CAD build for the part. Positions are in the model's coordinates, mm. A direction names the side the tool comes from. Coordinates: 2 decimals unless noted, no trailing zeros. Loops run counter-clockwise (first coordinate to the right, second up) from the corner with the lowest first, then second, coordinate; pieces in that order, holes last. Notation, with made-up numbers: (-33.5, 34) -> (20.5, 34) arc R15 ccw to (20.5, 48) -> close; hole circle Ø3 at (60.25, -32.5). An arc over 180 degrees is marked (long way). Return JSON: item names as keys, results as strings. Group by question number.
(1) Saw through at B-B on y = 0. Write the cut outline in (x, z).
(2) Saw through at D-D on x = 0. Write the cut outline in (y, z).
(3) Saw through at C-C on x = -8. Write the cut outline in (y, z), then the cut area to 3 significant figures.
(4) Probe L1, parallel to Y at x = 0, z = 24.7; L2, parallel to Y at x = -2, z = 63; L3, parallel to Z at x = 2, y = 3.5. List the from-to ranges inside material, lowest first.
(5) Flat gauge pins, fed straight in: pin 1 Ø21 at (y, z) = (8.5, 36.5) entering from -X; pin 2 Ø4 at (x, y) = (13, -8) entering from +Z; pin 3 Ø14.5 at (x, y) = (1, 1) entering from -Z; pin 4 Ø2 at (x, z) = (13, 26.5) entering from +Y. Where does each tip first touch, or does it go through?
(6) Saw through at A-A on z = 30. Write the cut outline in (x, y).
(7) Tool access for faces 1 (the face through (-7.64, -20.79, 57.59)), 2 (the face through (-14, 14, 0)), 3 (the face through (12, 0, 25)), 4 (the face through (4, 0, 24)): list every direction of +Z, -Z, +X, -X, +Y, -Y with a clear straight run to the whole face (end or side of a thin tool).
(8) Mould opens along X. For faces 5 (the face through (-15.16, -11.62, 11.83)), 6 (the face through (-4.39, -19.79, 12.32)), 7 (the face through (-6.5, 0, 27)) say: pulls with the +X half, pulls with the -X half, needs draft (parallel to the pull), parting line crosses it, or undercut.
```python
from build123d import *

# Parameters (mm, degrees)
F0_R      = 20.2700767199
F0_R_2    = 19.1
F0_R_3    = 2
F1_DEPTH  = 25
F2_DEPTH  = 24
F3_W      = 13
F3_H      = 13
F3_R      = 2
F4_DEPTH  = 3
F5_DEPTH  = 15
F6_DEPTH  = 15
F7_W      = 13
F7_H      = 2.5
F8_DEPTH  = 60
F9_W      = 13
F9_H      = 2.5
F10_DEPTH = 40
F11_W     = 2.5
F11_H     = 11.5
F11_W_2   = 2.3203180134
F12_DEPTH = 6
F13_W     = 2.5
F13_H     = 11.5
F14_DEPTH = 40
F15_W     = 2.5
F15_H     = 11.5
F16_DEPTH = 3.6
F18_R     = 1
F17_R     = 1
F19_DEPTH = 5


with BuildPart() as f1:
    # F0 (on Top) → F1 (new body)
    with BuildSketch(Plane.XY):
        Circle(F0_R)
        Circle(F0_R_2, mode=Mode.SUBTRACT)
        Circle(F0_R_2)
        Circle(F0_R_3, mode=Mode.SUBTRACT)
    extrude(amount=F1_DEPTH)

    # F0 (on Top) → F2 (cut)
    with BuildSketch(Plane.XY):
        Circle(F0_R_2)
        Circle(F0_R_3, mode=Mode.SUBTRACT)
    extrude(amount=F2_DEPTH, mode=Mode.SUBTRACT)

    # F3 (on face) → F4 (join)
    with BuildSketch(Plane.XY.offset(25)):
        Rectangle(F3_W, F3_H)
        Circle(F3_R, mode=Mode.SUBTRACT)
        Rectangle(F3_W, F3_H)
    extrude(amount=F4_DEPTH)

    # F5 (add): a face of the model
    f5_faces = [f1.faces().sort_by_distance(p)[0] for p in [
        (0, -6.5, 26.5),
    ]]
    extrude(f5_faces, amount=F5_DEPTH)

    # F6 (add): a face of the model
    f6_faces = [f1.faces().sort_by_distance(p)[0] for p in [
        (0, 6.5, 26.5),
    ]]
    extrude(f6_faces, amount=F6_DEPTH)

    # F7 (on face) → F8 (join)
    with BuildSketch(Plane.XY.offset(28)):
        with Locations((0, -20.25)):
            Rectangle(F7_W, F7_H)
        with Locations((0, 20.25)):
            Rectangle(F7_W, F7_H)
    extrude(amount=F8_DEPTH)

    # F9 (on face) → F10 (join)
    with BuildSketch(Plane.XZ.offset(-19)):
        with Locations((0, 86.75)):
            Rectangle(F9_W, F9_H)
    extrude(amount=F10_DEPTH)

    # F11 (on face) → F12 (join)
    with BuildSketch(Plane.YZ.offset(6.5)):
        with Locations((-20.25, 56.75)):
            Rectangle(F11_W, F11_H)
        with Locations((20.3398409933, 56.75)):
            Rectangle(F11_W_2, F11_H)
    extrude(amount=F12_DEPTH)

    # F13 (on face) → F14 (join)
    with BuildSketch(Plane(origin=(0, -19, 0), x_dir=(-1, 0, 0), z_dir=(0, 1, 0))):
        with Locations((-11.25, 56.75)):
            Rectangle(F13_W, F13_H)
    extrude(amount=F14_DEPTH)

    # F15 (on face) → F16 (join)
    with BuildSketch(Plane(origin=(-6.5, 0, 0), x_dir=(0, -1, 0), z_dir=(-1, 0, 0))):
        with Locations((20.25, 56.75)):
            Rectangle(F15_W, F15_H)
        with Locations((-20.25, 56.75)):
            Rectangle(F15_W, F15_H)
    extrude(amount=F16_DEPTH)

    # F18 (on face) + F17 (on face) → F19 (cut)
    with BuildSketch(Plane(origin=(-10.1, 0, 0), x_dir=(0, -1, 0), z_dir=(-1, 0, 0))):
        with Locations((20.25, 56.75)):
            Circle(F18_R)
    with BuildSketch(Plane(origin=(-10.1, 0, 0), x_dir=(0, -1, 0), z_dir=(-1, 0, 0))):
        with Locations((-20.2555917203, 56.75)):
            Circle(F17_R)
    extrude(amount=-F19_DEPTH, mode=Mode.SUBTRACT)


solid = f1.part
```
Geometry results:
{
 "1": {"outline": "(-20.27, 0) -> (-19.1, 0) -> (-19.1, 24) -> (-2, 24) -> (-2, 25) -> (2, 25) -> (2, 24) -> (19.1, 24) -> (19.1, 0) -> (20.27, 0) -> (20.27, 25) -> (6.5, 25) -> (6.5, 28) -> (-6.5, 28) -> (-6.5, 25) -> (-20.27, 25) -> close; (-6.5, 85.5) -> (6.5, 85.5) -> (6.5, 88) -> (-6.5, 88) -> close; (10, 51) -> (12.5, 51) -> (12.5, 62.5) -> (10, 62.5) -> close"},
 "2": {"outline": "(-21.5, 25) -> (-20.27, 25) -> (-20.27, 0) -> (-19.1, 0) -> (-19.1, 24) -> (-2, 24) -> (-2, 25) -> (2, 25) -> (2, 24) -> (19.1, 24) -> (19.1, 0) -> (20.27, 0) -> (20.27, 25) -> (21.5, 25) -> (21.5, 88) -> (-21.5, 88) -> close; hole (-19, 28) -> (19, 28) -> (19, 85.5) -> (-19, 85.5) -> close"},
 "3": {"outline": "(-21.5, 51) -> (-19, 51) -> (-19, 62.5) -> (-21.5, 62.5) -> close; (-18.62, 0) -> (-17.34, 0) -> (-17.34, 24) -> (17.34, 24) -> (17.34, 0) -> (18.62, 0) -> (18.62, 25) -> (-18.62, 25) -> close; (19, 51) -> (21.5, 51) -> (21.5, 62.5) -> (19, 62.5) -> close; hole circle Ø2 at (-20.25, 56.75); hole circle Ø2 at (20.26, 56.75)", "area": "150 mm²"},
 "4": {"L1": "-20.27 to -2, 2 to 20.27", "L2": "-21.5 to -19, 19 to 21.5", "L3": "24 to 28, 85.5 to 88"},
 "5": {"pin 1": "x = -6.5", "pin 2": "z = 62.5", "pin 3": "z = 24", "pin 4": "through"},
 "6": {"outline": "(-6.5, -21.5) -> (6.5, -21.5) -> (6.5, -19) -> (-6.5, -19) -> close; (-6.5, 19) -> (6.5, 19) -> (6.5, 21.5) -> (-6.5, 21.5) -> close"},
 "7": {"face 1": "-X", "face 2": "-Z, +X, -X, +Y, -Y", "face 3": "+X, +Y, -Y", "face 4": "-Z"},
 "8": {"face 5": "undercut", "face 6": "parting line crosses it", "face 7": "pulls with the -X half"}
}
